```python
from build123d import *

# Parameters (mm, degrees)
SKETCH_1_W          = 31
SKETCH_1_H          = 42
EXTRUDE_1_DEPTH     = 7
SKETCH_3_W          = 6.699750495
SKETCH_3_H          = 3.302693905
EXTRUDE_2_DEPTH     = 5
SKETCH_4_W          = 2.984504837
SKETCH_4_H          = 2.652893189
EXTRUDE_3_DEPTH     = 2
SKETCH_5_W          = 8
SKETCH_5_H          = 2.576224576
EXTRUDE_4_DEPTH     = 2
SKETCH_6_R          = 1.726982995
CUT_EXTRUDE_1_DEPTH = 8
SKETCH_7_W          = 5.173141718
SKETCH_7_H          = 4.77520774
SKETCH_7_W_2        = 13.421733696
SKETCH_7_H_2        = 3.175273919
EXTRUDE_5_DEPTH     = 3
SKETCH_8_W          = 0.5
SKETCH_8_H          = 0.5
EXTRUDE_6_DEPTH     = 4


with BuildPart() as part:
    # 草圖1 → 填料-伸長1 (new body)
    with BuildSketch(Plane(origin=(0, 0, 0), x_dir=(1, 0, 0), z_dir=(0, 1, 0))):
        with Locations((15.5, 21)):
            Rectangle(SKETCH_1_W, SKETCH_1_H)
    extrude(amount=EXTRUDE_1_DEPTH)

    # 草圖3 → 填料-伸長2 (add)
    with BuildSketch(Plane(origin=(0, 7, 0), x_dir=(1, 0, 0), z_dir=(0, 1, 0))):
        with Locations((15.108684373, 38.694954661)):
            Rectangle(SKETCH_3_W, SKETCH_3_H)
        with Locations((5.108684373, 38.694954661)):
            Rectangle(SKETCH_3_W, SKETCH_3_H)
        with Locations((25.108684373, 38.694954661)):
            Rectangle(SKETCH_3_W, SKETCH_3_H)
    extrude(amount=EXTRUDE_2_DEPTH)

    # 草圖4 → 填料-伸長3 (add)
    with BuildSketch(Plane(origin=(0, 7, 0), x_dir=(1, 0, 0), z_dir=(0, 1, 0))):
        with Locations((7.315015434, 34.091646646)):
            Rectangle(SKETCH_4_W, SKETCH_4_H)
        with Locations((2.315015434, 34.091646646)):
            Rectangle(SKETCH_4_W, SKETCH_4_H)
        with Locations((12.315015434, 34.091646646)):
            Rectangle(SKETCH_4_W, SKETCH_4_H)
        with Locations((17.315015434, 34.091646646)):
            Rectangle(SKETCH_4_W, SKETCH_4_H)
        with Locations((22.315015434, 34.091646646)):
            Rectangle(SKETCH_4_W, SKETCH_4_H)
        with Locations((27.315015434, 34.091646646)):
            Rectangle(SKETCH_4_W, SKETCH_4_H)
    extrude(amount=EXTRUDE_3_DEPTH)

    # 草圖5 → 填料-伸長4 (add)
    with BuildSketch(Plane(origin=(0, 7, 0), x_dir=(1, 0, 0), z_dir=(0, 1, 0))):
        with Locations((15.5, 28.828363784)):
            Rectangle(SKETCH_5_W, SKETCH_5_H)
    extrude(amount=EXTRUDE_4_DEPTH)

    # 草圖6 → 除料-伸長1 (cut, through all)
    with BuildSketch(Plane(origin=(0, 7, 0), x_dir=(1, 0, 0), z_dir=(0, 1, 0))):
        with Locations((2.25, 29.011078955)):
            Circle(SKETCH_6_R)
        with Locations((28.75, 29.011078955)):
            Circle(SKETCH_6_R)
    extrude(amount=-CUT_EXTRUDE_1_DEPTH, mode=Mode.SUBTRACT)

    # 草圖7 → 填料-伸長5 (add)
    with BuildSketch(Plane(origin=(0, 7, 0), x_dir=(1, 0, 0), z_dir=(0, 1, 0))):
        with Locations((15.187222404, 19.232590782)):
            Rectangle(SKETCH_7_W, SKETCH_7_H)
        with Locations((4.187222404, 19.232590782)):
            Rectangle(SKETCH_7_W, SKETCH_7_H)
        with Locations((26.187222404, 19.232590782)):
            Rectangle(SKETCH_7_W, SKETCH_7_H)
        with Locations((15.263552758, 1.58763696)):
            Rectangle(SKETCH_7_W_2, SKETCH_7_H_2)
    extrude(amount=EXTRUDE_5_DEPTH)

    # 草圖8 → 填料-伸長6 (add)
    with BuildSketch(Plane.XY):
        with Locations((9.895624486, 9.75)):
            Rectangle(SKETCH_8_W, SKETCH_8_H)
        with Locations((12.395624486, 9.75)):
            Rectangle(SKETCH_8_W, SKETCH_8_H)
        with Locations((14.895624486, 9.75)):
            Rectangle(SKETCH_8_W, SKETCH_8_H)
        with Locations((17.395624486, 9.75)):
            Rectangle(SKETCH_8_W, SKETCH_8_H)
        with Locations((19.895624486, 9.75)):
            Rectangle(SKETCH_8_W, SKETCH_8_H)
    extrude(amount=EXTRUDE_6_DEPTH)


solid = part.part
```
Check sheet for the modelled part. Datum: model origin and axes. Units: mm. A direction names the side the tool comes from. Round coordinates to 2 decimals unless told otherwise and drop trailing zeros. Write each loop counter-clockwise with the first axis right and the second up, starting at its lowest first coordinate (ties: lowest second). Pieces come first, ordered by that corner, then holes. Notation, with made-up numbers: (78, -25.5) -> (136, -25.5) arc R11 ccw to (136, -9.5) -> close; hole circle Ø11 at (-22.75, -31.75). An arc over 180 degrees is marked (long way). One line per question, with ' | ' between items. Start each with the question number.
1. Sectioned sample at D-D, the plane z = -25.5. Record the cut outline in (x, y).
2. Scan lines: line 1 along X through (y, z) = (8.5, -17); line 2 along X through (y, z) = (10.25, -38); line 3 along X through (y, z) = (9.75, 1). Record each from-to range of solid material in increasing order. Write a range as from..to.
3. Sectioned sample at A-A, the plane x = 2.25. Record the cut outline in (y, z).
4. Set-up check for faces 4 (the face through (15, 10, -19)), 5 (the face through (20.823, 8, -34)), 6 (the face through (13.807, 8, -34)), 7 (the face through (5, 9, -37.044)): record each of +Z, -Z, +X, -X, +Y, -Y from which the full face is reachable in a straight line by a thin tool's end or side.
5. Sectioned sample at C-C, the plane x = 7.5. Record the cut outline in (y, z), then the cut area to 3 significant figures.
6. Release check for a two-part mould opening along Z. For faces 1 (the face through (25, 9, -40.346)), 2 (the face through (8.807, 8, -34)), 3 (the face through (2, 9, -34)) record: +Z half, -Z half, draft (parallel to the pull), parting line (faces both ways), or undercut.
7. Sectioned sample at B-B, the plane z = -33.5. Record the cut outline in (x, y).
8. Depth check by flat-ended pin: pin 1 (0.6 mm diameter, centred on x = 8, y = 8, fed in from +Z); pin 2 (0.9 mm diameter, centred on y = 8, z = -20, fed in from -X); pin 3 (3 mm diameter, centred on x = 6, z = -27.5, fed in from +Y); pin 4 (3 mm diameter, centred on x = 2.25, z = -29.01, fed in from -Y). Enter the tip coordinate at first touch or a pass-through.
Taken from the geometry:
1) outline: (0, 0) -> (31, 0) -> (31, 7) -> (0, 7) -> close
2) line 1: x = 1.6..6.77, 12.6..17.77, 23.6..28.77 | line 2: x = 1.76..8.46, 11.76..18.46, 21.76..28.46 | line 3: x = 9.65..10.15, 12.15..12.65, 14.65..15.15, 17.15..17.65, 19.65..20.15
3) outline: (0, -42) -> (7, -42) -> (7, -40.35) -> (12, -40.35) -> (12, -37.04) -> (7, -37.04) -> (7, -35.42) -> (9, -35.42) -> (9, -32.77) -> (7, -32.77) -> (7, -30.74) -> (0, -30.74) -> close; (0, -27.28) -> (7, -27.28) -> (7, -21.62) -> (10, -21.62) -> (10, -16.84) -> (7, -16.84) -> (7, 0) -> (0, 0) -> close
4) face 4: +Z, +X, -X, +Y | face 5: -Z, +Y | face 6: +Y | face 7: +X, -X, +Y
5) outline: (0, -42) -> (7, -42) -> (7, -40.35) -> (12, -40.35) -> (12, -37.04) -> (7, -37.04) -> (7, -35.42) -> (9, -35.42) -> (9, -32.77) -> (7, -32.77) -> (7, 0) -> (0, 0) -> close | area: 316 mm^2
6) face 1: -Z half | face 2: draft | face 3: undercut
7) outline: (0, 0) -> (31, 0) -> (31, 7) -> (28.81, 7) -> (28.81, 9) -> (25.82, 9) -> (25.82, 7) -> (23.81, 7) -> (23.81, 9) -> (20.82, 9) -> (20.82, 7) -> (18.81, 7) -> (18.81, 9) -> (15.82, 9) -> (15.82, 7) -> (13.81, 7) -> (13.81, 9) -> (10.82, 9) -> (10.82, 7) -> (8.81, 7) -> (8.81, 9) -> (5.82, 9) -> (5.82, 7) -> (3.81, 7) -> (3.81, 9) -> (0.82, 9) -> (0.82, 7) -> (0, 7) -> close
8) pin 1: stops at z = -32.77 | pin 2: stops at x = 1.6 | pin 3: stops at y = 7 | pin 4: passes through
